from build123d import *

# Parameters (mm, degrees)
EXTRUDE_1_DEPTH = 18


with BuildPart() as part:
    # 草图1 → 凸台-拉伸1 (new body)
    with BuildSketch(Plane.XY):
        with BuildLine():
            Line((5, 4.5), (5, 19.5))
            Line((5, 19.5), (9.25, 19.5))
            ThreePointArc((9.25, 19.5), (10, 18.75), (9.25, 18))
            ThreePointArc((9.25, 18), (8.5, 17.25), (9.25, 16.5))
            ThreePointArc((9.25, 16.5), (10, 15.75), (9.25, 15))
            ThreePointArc((9.25, 15), (8.5, 14.25), (9.25, 13.5))
            ThreePointArc((9.25, 13.5), (10, 12.75), (9.25, 12))
            ThreePointArc((9.25, 12), (8.5, 11.25), (9.25, 10.5))
            ThreePointArc((9.25, 10.5), (10, 9.75), (9.25, 9))
            ThreePointArc((9.25, 9), (8.5, 8.25), (9.25, 7.5))
            ThreePointArc((9.25, 7.5), (10, 6.75), (9.25, 6))
            ThreePointArc((9.25, 6), (8.5, 5.25), (9.25, 4.5))
            ThreePointArc((9.25, 4.5), (10, 3.75), (9.25, 3))
            ThreePointArc((9.25, 3), (8.5, 2.25), (9.25, 1.5))
            ThreePointArc((9.25, 1.5), (10, 0.75), (9.25, 0))
            Line((9.25, 0), (0, 0))
            Line((0, 0), (0, 4.5))
            Line((0, 4.5), (5, 4.5))
        make_face()
    extrude(amount=EXTRUDE_1_DEPTH)


solid = part.part
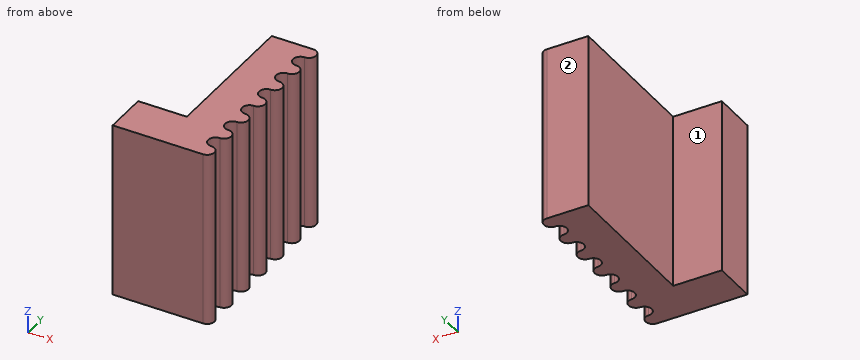
Build history of the part. All positions in model axes, mm. Face numbers are marked on the shaded views. A direction names the side the tool comes from. Coordinates: 2 decimals unless noted, no trailing zeros. Write each loop counter-clockwise with the first axis right and the second up, starting at its lowest first coordinate (ties: lowest second). Pieces come first, ordered by that corner, then holes.
(1) Cut at A-A on x = 9. List the corners of the cut face in (y, z).
(2) Drill centre lines: line 1 (Y direction, x = 2.75, z = 5.25); line 2 (X direction, y = 8.25, z = 12.5); line 3 (X direction, y = 10.75, z = 12.5). Where is each one in solid material? Low to high.
(3) Cut at B-B on z = 15.5. List the corners of the cut face in (x, y).
(4) 3-axis set-ups, long thin cutter, end or side, ignore diameter. For the marked faces 1 and 2: which of +Z, -Z, +X, -X, +Y, -Y reach the whole face in a straight line?
(5) Cut at D-D on x = 2. List the corners of the cut face in (y, z).
(6) Pin check, flat tip, straight feed: pin 1 Ø7.5 at (y, z) = (14.5, 8) entering from -X. Stop position of the tip, or through.
(7) Cut at C-C on y = 9.75. List the corners of the cut face in (x, z).
Working result:
1. outline: (0, 0) - (1.54, 0) - (1.54, 18) - (0, 18) - close; (2.96, 0) - (4.54, 0) - (4.54, 18) - (2.96, 18) - close; (5.96, 0) - (7.54, 0) - (7.54, 18) - (5.96, 18) - close; (8.96, 0) - (10.54, 0) - (10.54, 18) - (8.96, 18) - close; (11.96, 0) - (13.54, 0) - (13.54, 18) - (11.96, 18) - close; (14.96, 0) - (16.54, 0) - (16.54, 18) - (14.96, 18) - close; (17.96, 0) - (19.5, 0) - (19.5, 18) - (17.96, 18) - close
2. line 1: y = 0 to 4.5
2. line 2: x = 5 to 8.5
2. line 3: x = 5 to 8.69
3. outline: (0, 0) - (9.25, 0) arc R0.75 ccw to (9.25, 1.5) arc R0.75 cw to (9.25, 3) arc R0.75 ccw to (9.25, 4.5) arc R0.75 cw to (9.25, 6) arc R0.75 ccw to (9.25, 7.5) arc R0.75 cw to (9.25, 9) arc R0.75 ccw to (9.25, 10.5) arc R0.75 cw to (9.25, 12) arc R0.75 ccw to (9.25, 13.5) arc R0.75 cw to (9.25, 15) arc R0.75 ccw to (9.25, 16.5) arc R0.75 cw to (9.25, 18) arc R0.75 ccw to (9.25, 19.5) - (5, 19.5) - (5, 4.5) - (0, 4.5) - close
4. face 1: +Z, -Z, -X, +Y
4. face 2: +Z, -Z, +X, -X, +Y
5. outline: (0, 0) - (4.5, 0) - (4.5, 18) - (0, 18) - close
6. pin 1: stops at x = 5
7. outline: (5, 0) - (10, 0) - (10, 18) - (5, 18) - close
